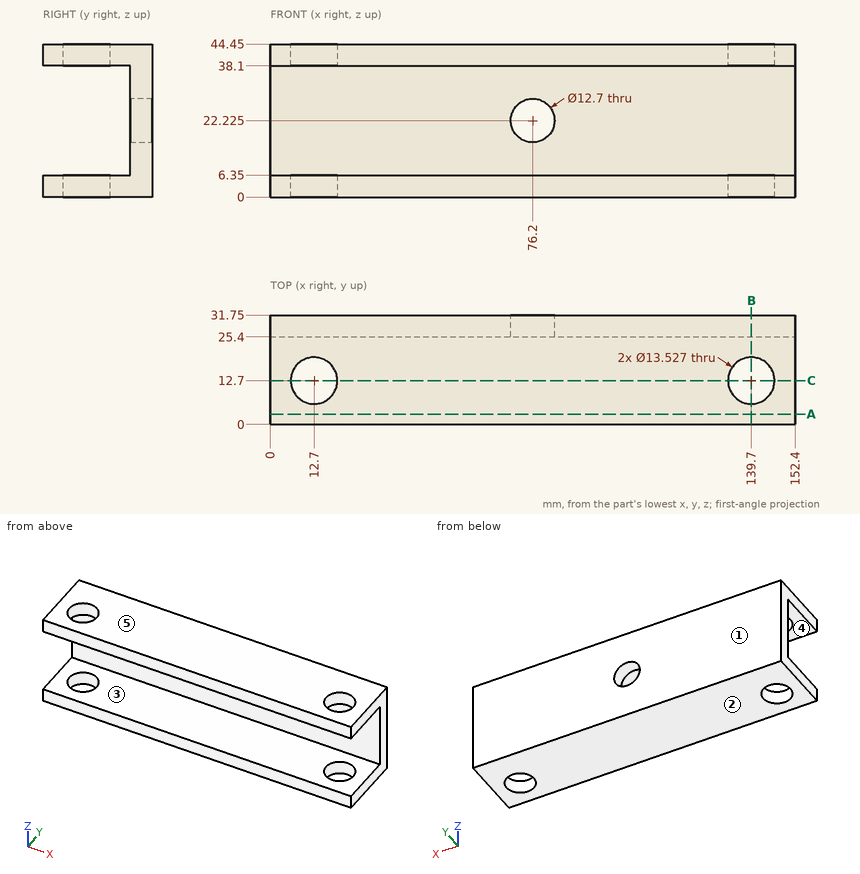
Could you check a few things on this drawing? It's one solid part, dimensions in mm from its lowest x, y, z. A direction names the side the tool comes from. Coordinates: 2 decimals unless noted, no trailing zeros. Write each loop counter-clockwise with the first axis right and the second up, starting at its lowest first coordinate (ties: lowest second). Pieces come first, ordered by that corner, then holes. Notation, with made-up numbers: (55, 36) - (99, 36) arc R29 ccw to (99, 65) - close; hole circle Ø5 at (77, 79.25). An arc over 180 degrees is marked (long way). Return JSON: item names as keys, results as strings. Group by question number.
Item 1: Please list where these lines run through material, in increasing order: probe 1 along Y at (x, z) = (12.7, 4.25); probe 2 along Z at (x, y) = (69, 14); probe 3 along X at (y, z) = (12, 3).
Item 2: Which directions (+Z, -Z, +X, -X, +Y, -Y) give clear straight access to the entire face, cutting with the end or side of a thin tool? Please do the marked faces 4 and 5.
Item 3: If we section it at B-B (x = 139.7): Write out the boundary of the cut face in (y, z).
Item 4: If we section it at A-A (y = 3): Write out the boundary of the cut face in (x, z).
Item 5: We'd pull the mould along Z, two halves only. Please class the marked faces 1, 2 and 3: pulls with the +Z half, pulls with the -Z half, needs draft (parallel to the pull), parting line crosses it, or undercut.
Item 6: If we section it at C-C (y = 12.7): Write out the boundary of the cut face in (x, z), then the cut area to 3 significant figures.
Item 7: I'm going to push flat-ended pins straight in: pin 1 Ø12 at (x, y) = (12.7, 12.7) entering from -Z; pin 2 Ø12 at (x, z) = (46.5, 27.5) entering from -Y. Where does each tip first touch, or does it pass through?
Return value:
{
 "1": {"probe 1": "y = 0 to 5.94, 19.46 to 31.75", "probe 2": "z = 0 to 6.35, 38.1 to 44.45", "probe 3": "x = 0 to 5.97, 19.43 to 132.97, 146.43 to 152.4"},
 "2": {"face 4": "+X, -X, -Y", "face 5": "+Z, +X, -X, +Y, -Y"},
 "3": {"outline": "(0, 0) - (5.94, 0) - (5.94, 6.35) - (0, 6.35) - close; (0, 38.1) - (5.94, 38.1) - (5.94, 44.45) - (0, 44.45) - close; (19.46, 0) - (31.75, 0) - (31.75, 44.45) - (19.46, 44.45) - (19.46, 38.1) - (25.4, 38.1) - (25.4, 6.35) - (19.46, 6.35) - close"},
 "4": {"outline": "(0, 0) - (152.4, 0) - (152.4, 6.35) - (0, 6.35) - close; (0, 38.1) - (152.4, 38.1) - (152.4, 44.45) - (0, 44.45) - close"},
 "5": {"face 1": "needs draft", "face 2": "pulls with the -Z half", "face 3": "undercut"},
 "6": {"outline": "(0, 0) - (5.94, 0) - (5.94, 6.35) - (0, 6.35) - close; (0, 38.1) - (5.94, 38.1) - (5.94, 44.45) - (0, 44.45) - close; (19.46, 0) - (132.94, 0) - (132.94, 6.35) - (19.46, 6.35) - close; (19.46, 38.1) - (132.94, 38.1) - (132.94, 44.45) - (19.46, 44.45) - close; (146.46, 0) - (152.4, 0) - (152.4, 6.35) - (146.46, 6.35) - close; (146.46, 38.1) - (152.4, 38.1) - (152.4, 44.45) - (146.46, 44.45) - close", "area": "1,590 mm^2"},
 "7": {"pin 1": "passes through", "pin 2": "stops at y = 25.4"}
}
